```python
from build123d import *

# Parameters (mm, degrees)
BOSS_EXTRUDE1_DEPTH = 15
FILLET1_R           = 20
FILLET2_R           = 15
SKETCH2_W           = 5
SKETCH2_H           = 60
CUT_EXTRUDE1_DEPTH  = 24


with BuildPart() as part:
    # Sketch1 → Boss-Extrude1 (new body)
    # profile 1 of 6: a face of its own
    with BuildSketch(Plane.XY):
        with BuildLine():
            Line((-20, -30), (-30, -30))
            ThreePointArc((-30, -30), (-29.388396861, -36.026784376), (-27.578524672, -41.807835403))
            Line((-27.578524672, -41.807835403), (-20, -30))
        make_face()
    # profile 2 of 6: a face of its own
    with BuildSketch(Plane.XY):
        with BuildLine():
            Line((0, -10), (0, 0))
            ThreePointArc((0, 0), (-21.213203436, -8.786796564), (-30, -30))
            Line((-30, -30), (-20, -30))
            ThreePointArc((-20, -30), (-14.142135624, -15.857864376), (0, -10))
        make_face()
    # profile 3 of 6: a face of its own
    with BuildSketch(Plane.XY):
        with BuildLine():
            ThreePointArc((0, -50), (-14.142135624, -44.142135624), (-20, -30))
            Line((-20, -30), (-27.578524672, -41.807835403))
            ThreePointArc((-27.578524672, -41.807835403), (-16.519154608, -55.04231481), (0, -60))
            Line((0, -60), (0, -50))
        make_face()
    # profile 4 of 6: a face of its own
    with BuildSketch(Plane.XY):
        with BuildLine():
            ThreePointArc((-27.578524672, -41.807835403), (-29.388396861, -36.026784376), (-30, -30))
            Line((-30, -30), (-49.254650189, -60))
            Line((-49.254650189, -60), (-30, -105))
            ThreePointArc((-30, -105), (-28.650020621, -98.780921528), (-24.84307506, -93.681260081))
            Line((-24.84307506, -93.681260081), (-39.254650189, -60))
            Line((-39.254650189, -60), (-27.578524672, -41.807835403))
        make_face()
    # profile 5 of 6: a face of its own
    with BuildSketch(Plane.XY):
        with BuildLine():
            ThreePointArc((-24.84307506, -93.681260081), (-28.650020621, -98.780921528), (-30, -105))
            Line((-30, -105), (-20, -105))
            Line((-20, -105), (-24.84307506, -93.681260081))
        make_face()
    # profile 6 of 6: a face of its own
    with BuildSketch(Plane.XY):
        with BuildLine():
            Line((-20, -105), (-30, -105))
            ThreePointArc((-30, -105), (-15, -120), (0, -105))
            ThreePointArc((0, -105), (-8.780921528, -91.349979379), (-24.84307506, -93.681260081))
            Line((-24.84307506, -93.681260081), (-20, -105))
        make_face()
        with BuildLine():
            ThreePointArc((-10, -105), (-15, -110), (-20, -105))
            ThreePointArc((-20, -105), (-15, -100), (-10, -105))
        make_face(mode=Mode.SUBTRACT)
    extrude(amount=BOSS_EXTRUDE1_DEPTH)

    # Fillet1
    fillet1_edges = [part.edges().sort_by_distance(p)[0] for p in [
        (-39.254650189, -60, 7.5),
        (-49.254650189, -60, 7.5),
    ]]
    fillet(fillet1_edges, radius=FILLET1_R)

    # Fillet2
    # the kernel refuses this fillet: 15 mm, written as the material it takes off along each edge
    with BuildSketch(Plane(origin=(0, -50, -25), x_dir=(-0.9759000729485309, 0.21821789023600283, 0), z_dir=(0, 0, 1))) as fillet2_piece_1:
        with BuildLine():
            CenterArc((12.001983963, 14.638501094), FILLET2_R, 198.983752857, 58.411864495)
            Line((-2.182178902, 9.759000729), (-2.46586216, 9.661410722))
            ThreePointArc((-2.46586216, 9.661410722), (-1.383859473, 4.814034998), (-0.292770022, -0.065465367))
            Line((-0.292770022, -0.065465367), (0.065465367, -0.292770022))
            ThreePointArc((0.065465367, -0.292770022), (4.364357805, 0.181998541), (8.663250242, -0.292770022))
            Line((8.663250242, -0.292770022), (8.728715609, 0))
        make_face()
    extrude(amount=65, mode=Mode.SUBTRACT)
    with BuildSketch(Plane(origin=(0, -10, -25), x_dir=(0, 1, 0), z_dir=(0, 0, 1))) as fillet2_piece_2:
        with BuildLine():
            CenterArc((11.666666667, 14.90711985), FILLET2_R, 205.208765297, 58.411864495)
            Line((-1.904761905, 8.5183542), (-2.176190476, 8.390578887))
            ThreePointArc((-2.176190476, 8.390578887), (-0.774768563, 4.298892438), (-0.3, 0))
            Line((-0.3, 0), (0, -0.3))
            ThreePointArc((0, -0.3), (5, -0.3), (9.966666667, -0.298142397))
            Line((9.966666667, -0.298142397), (10, 0))
        make_face()
    extrude(amount=65, mode=Mode.SUBTRACT)

    # Sketch2 → Cut-Extrude1 (cut)
    with BuildSketch(Plane(origin=(0, 0, 0), x_dir=(0, 0, -1), z_dir=(1, 0, 0))):
        with Locations((-7.5, -30)):
            Rectangle(SKETCH2_W, SKETCH2_H)
    extrude(amount=-CUT_EXTRUDE1_DEPTH, mode=Mode.SUBTRACT)


solid = part.part
```
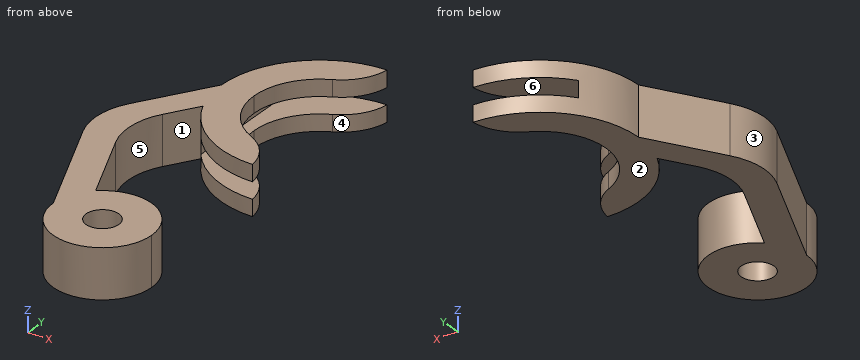
Check sheet for the modelled part. Datum: model origin and axes. Units: mm. Face numbers are marked on the shaded views. A direction names the side the tool comes from. Give positions to 0.01 mm unless a question says otherwise; leave off trailing zeros. Write each loop counter-clockwise with the first axis right and the second up, starting at its lowest first coordinate (ties: lowest second). Pieces come first, ordered by that corner, then holes.
Item 1: Cross-section at D-D (y = -16). Enter the section's corners in (x, z), and give its area (3 significant figures).
Item 2: Cross-section at C-C (x = -3.5). Enter the section's corners in (y, z).
Item 3: Gauge pin test, flat ends, axial feed: pin 1 (1.5 mm diameter, centred on y = -23, z = 6.5, fed in from +X); pin 2 (2 mm diameter, centred on y = -67.5, z = 13, fed in from +X); pin 3 (2 mm diameter, centred on x = -35.5, z = 3, fed in from +Y). Record the tip position at first contact, or that the pin passes through.
Item 4: Draft check along X on the marked faces 1, 2 and 3. Enter one of: released by +X, released by -X, zero draft, split by the parting line, or undercut.
Item 5: Access from +Z, -Z, +X, -X, +Y, -Y to the whole of each face (thin tool, end or side, straight path). Record for the marked faces 4, 5 and 6.
Item 6: Cross-section at B-B (x = -32). Enter the section's corners in (y, z), and give its area (3 significant figures).
Item 7: Scan lines: L1, parallel to Z at x = -8, y = -49.5; L2, parallel to Y at x = -15, z = 9.25; L3, parallel to Y at x = -15, z = 10.5. Record each from-to range of solid material in increasing order.
Item 8: Cross-section at A-A (z = 12.5). Enter the section's corners in (x, y), and give its area (3 significant figures).
Report:
1. outline: (-26.53, 0) - (-14.28, 0) - (-14.28, 5) - (-24, 5) - (-24, 10) - (-14.28, 10) - (-14.28, 15) - (-26.53, 15) - close
1. area: 135 mm2
2. outline: (-114.63, 0) - (-95.37, 0) - (-95.37, 15) - (-114.63, 15) - close; (-59.8, 0) - (-51.93, 0) - (-51.93, 5) - (-59.8, 5) - close; (-59.8, 10) - (-51.93, 10) - (-51.93, 15) - (-59.8, 15) - close; (-8.07, 0) - (-0.2, 0) - (-0.2, 5) - (-8.07, 5) - close; (-8.07, 10) - (-0.2, 10) - (-0.2, 15) - (-8.07, 15) - close
3. pin 1: stops at x = -24
3. pin 2: stops at x = -35.57
3. pin 3: stops at y = -37.01
4. face 1: undercut
4. face 2: zero draft
4. face 3: released by -X
5. face 4: +Z, -Z, +X
5. face 5: +Z, -Z
5. face 6: +X, +Y
6. outline: (-100.33, 0) - (-76.95, 0) - (-76.95, 15) - (-100.33, 15) - close; (-48.7, 0) - (-33.12, 0) - (-33.12, 15) - (-48.7, 15) - close
6. area: 584 mm2
7. L1: z = 0 to 5, 10 to 15
7. L2: y = -120 to -110, -100 to -90
7. L3: y = -120 to -110, -100 to -90, -55.98 to -43.23, -16.77 to -4.02
8. outline: (-45.08, -69.75) - (-30, -105) arc R15 ccw (long way) to (-24.84, -93.68) - (-35.08, -69.75) arc R20 cw to (-33.53, -51.08) - (-27.58, -41.81) arc R30 ccw to (0, -60) arc R15 ccw to (-8.52, -48.1) arc R20 cw to (-8.52, -11.9) arc R15 ccw to (0, 0) arc R30 ccw to (-30, -30) - (-43.53, -51.08) arc R20 ccw to start; hole circle Ø10 at (-15, -105)
8. area: 1,990 mm2
